Input: part model. Units: mm. Frame: model coordinates. Face numbers are marked on the shaded views. A direction names the side the tool comes from. Give positions to 0.01 mm unless a question says otherwise; leave off trailing zeros. Write each loop counter-clockwise with the first axis right and the second up, starting at its lowest first coordinate (ties: lowest second). Pieces come first, ordered by that corner, then holes.
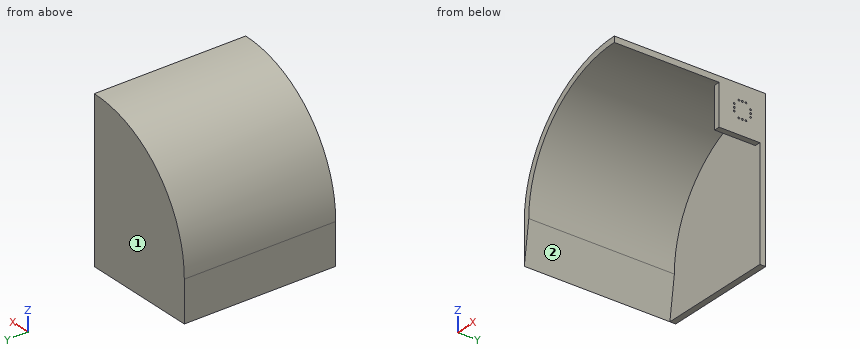
```python
from build123d import *

# Parameters (mm, degrees)
BOSS_EXTRUDE1_DEPTH = 130
CUT_EXTRUDE1_DEPTH  = 125
SKETCH7_W           = 35
SKETCH7_H           = 35
BOSS_EXTRUDE3_DEPTH = 5
SKETCH8_R           = 0.75
CUT_EXTRUDE2_DEPTH  = 5


with BuildPart() as part:
    # Sketch2 → Boss-Extrude1 (new body)
    with BuildSketch(Plane(origin=(0, 0, 0), x_dir=(1, 0, 0), z_dir=(0, 1, 0))):
        with BuildLine():
            Line((0, -100), (0, 35))
            Line((0, 35), (-100, 35))
            Line((-100, 35), (-100, 0))
            ThreePointArc((-100, 0), (-70.710678119, -70.710678119), (0, -100))
        make_face()
    extrude(amount=BOSS_EXTRUDE1_DEPTH)

    # Sketch3 → Cut-Extrude1 (cut)
    with BuildSketch(Plane.XZ):
        with BuildLine():
            Line((0, 95), (0, -35))
            Line((0, -35), (-100, -35))
            Line((-100, -35), (-95, 0))
            ThreePointArc((-95, 0), (-67.175144213, 67.175144213), (0, 95))
        make_face()
    extrude(amount=-CUT_EXTRUDE1_DEPTH, mode=Mode.SUBTRACT)

    # Sketch7 → Boss-Extrude3 (add)
    with BuildSketch(Plane(origin=(0, 0, 0), x_dir=(0, 0, -1), z_dir=(1, 0, 0))):
        with Locations((-77.5, 107.5)):
            Rectangle(SKETCH7_W, SKETCH7_H)
    extrude(amount=-BOSS_EXTRUDE3_DEPTH)

    # Sketch8 → Cut-Extrude2 (cut)
    with BuildSketch(Plane(origin=(0, 0, 0), x_dir=(0, 0, -1), z_dir=(1, 0, 0))):
        with Locations((-87, 110)):
            Circle(SKETCH8_R)
        with Locations((-87, 107)):
            Circle(SKETCH8_R)
        with Locations((-87, 113)):
            Circle(SKETCH8_R)
        with Locations((-77, 117)):
            Circle(SKETCH8_R)
        with Locations((-80, 117)):
            Circle(SKETCH8_R)
        with Locations((-83, 117)):
            Circle(SKETCH8_R)
        with Locations((-73, 107)):
            Circle(SKETCH8_R)
        with Locations((-73, 110)):
            Circle(SKETCH8_R)
        with Locations((-73, 113)):
            Circle(SKETCH8_R)
        with Locations((-83, 103)):
            Circle(SKETCH8_R)
        with Locations((-80, 103)):
            Circle(SKETCH8_R)
        with Locations((-77, 103)):
            Circle(SKETCH8_R)
    extrude(amount=-CUT_EXTRUDE2_DEPTH, mode=Mode.SUBTRACT)


solid = part.part
```
Item 1: Ray query, line 1 (Y direction, x = -1.45, z = 80); line 2 (Z direction, x = -2, y = 110); line 3 (Y direction, x = -1.8, z = 73). Return the intervals inside material, ascending.
Item 2: Section A-A (y = 100.5). Return loops of the section in (x, z), and give its area (3 significant figures).
Item 3: Set-up query: the marked faces 1 and 2. Return all of +Z, -Z, +X, -X, +Y, -Y with unobstructed straight access to the full face (end or side cutting, diameter ignored); none if empty.
Item 4: Section D-D (y = 61.5). Return loops of the section in (x, z).
Item 5: Section B-B (x = -84.5). Return loops of the section in (y, z).
Item 6: Pin query (flat end, axial travel): pin 1 (2.5 mm diameter, centred on y = 103, z = 77, fed in from -X); pin 2 (1.2 mm diameter, centred on y = 107, z = 73, fed in from +X); pin 3 (2 mm diameter, centred on y = 56, z = 33.5, fed in from +X). Return the tip coordinate at first contact, or that it passes through.
Item 7: Section C-C (z = -22.5). Return loops of the section in (x, y), and give its area (3 significant figures).
Solved:
1. line 1: y = 90 to 102.25, 103.75 to 116.25, 117.75 to 130
1. line 2: z = 60 to 72.25, 73.75 to 86.25, 87.75 to 99.98
1. line 3: y = 90 to 106.25, 107.75 to 109.25, 110.75 to 112.25, 113.75 to 130
2. outline: (-100, -35) - (-95, 0) arc R95 cw to (-5, 94.87) - (-5, 60) - (0, 60) - (0, 100) arc R100 ccw to (-100, 0) - close
2. area: 1,030 mm2
3. face 1: +Z, -Z, +X, -X, +Y
3. face 2: -Z, +X, -Y
4. outline: (-100, -35) - (-95, 0) arc R95 cw to (0, 95) - (0, 100) arc R100 ccw to (-100, 0) - close
5. outline: (0, 43.41) - (125, 43.41) - (125, -35) - (130, -35) - (130, 53.48) - (0, 53.48) - close
6. pin 1: stops at x = -65.28
6. pin 2: stops at x = -60.07
6. pin 3: stops at x = -88.51
7. outline: (-100, 0) - (-98.21, 0) - (-98.21, 125) - (0, 125) - (0, 130) - (-100, 130) - close
7. area: 723 mm2
